Autodesk Inventor part; units mm, degrees
ref_plane "Work Plane8" through (0, 26.3, 0) normal (0, 1, 0) x (1, 0, 0)
ref_plane "Work Plane9" through (0, 30.1, 0) normal (0, 1, 0) x (1, 0, 0)
ref_plane "Work Plane15" through (-1.25, 15.4, 2.1651) normal (-0.5, 0, 0.866) x (0, -1, 0)
sketch "Sketch1" plane through (0, 0, 0) normal (1, 0, 0) x (0, 1, 0)
  line L0 (32, 0) -> (32, 2.45)
  line L1 (32, 2.45) -> (30.5, 2.45)
  line L2 (30.5, 2.45) -> (30.5, 2.125)
  line L3 (30.5, 2.125) -> (29.7, 2.125)
  line L4 (29.7, 2.125) -> (29.7, 2.45)
  line L5 (29.7, 2.45) -> (26.7, 2.45)
  line L6 (26.7, 2.45) -> (26.7, 2.125)
  line L7 (26.7, 2.125) -> (25.9, 2.125)
  line L8 (25.9, 2.125) -> (25.9, 2.45)
  line L9 (25.9, 2.45) -> (24.4, 2.45)
  line L10 (23.4, 2.5) -> (24.4, 2.5)
  line L11 (24.4, 2.5) -> (24.4, 2.45)
  line L12 (23.4, 2.5) -> (23.4, 7.5)
  line L13 (32, 2.45) -> (31, 2.45)
  line L14 (32, 2.45) -> (32, 1.45)
  line L15 (23.4, 7.5) -> (15.4, 7.5)
  line L16 (15.4, 7.5) -> (15.4, 0)
  line L17 (32, 0) -> (15.4, 0)
  point P0 (0, 0)
  dimension "d345" = 1.5
  dimension "d346" = 0.325
  dimension "d347" = 0.8
  dimension "d348" = 3
  dimension "d349" = 0.325
  dimension "d350" = 0.8
  dimension "d353" = 1
  dimension "d354" = 1
  dimension "d355" = 1
  dimension "d401" = 8
  dimension "d402" = 16.6
revolve "Revolution1" add sketch "Sketch1" angle 360 about axis through (0, 32, 0) along (0, -1, 0)
chamfer "Chamfer8" distance 1 angle 45 1 edges at (0, 32, -2.45)
sketch "Sketch13" plane through (0, 32, 0) normal (0, 1, 0) x (1, 0, 0)
  circle A0 centre (0, 0) radius 1
  point P0 (0, 0)
  dimension "d359" = 2
hole "Hole10" at (0, 32, 0) direction (0, -1, 0) diameter 2 end through all
ref_plane "Work Plane8" through (0, 26.3, 0) normal (0, 1, 0) x (1, 0, 0)
ref_plane "Work Plane9" through (0, 30.1, 0) normal (0, 1, 0) x (1, 0, 0)
sketch "Sketch16" plane through (0, 15.4, 0) normal (0, -1, 0) x (1, 0, 0)
  circle A0 centre (0, 0) radius 2.55
  dimension "d404" = 5.1
hole "Hole12" at (0, 15.4, 0) direction (0, 1, 0) diameter 5.1 depth 5
sketch "Sketch19" plane through (0, 15.4, 0) normal (0, -1, 0) x (1, 0, 0)
  circle A0 centre (0, 0) radius 7.5
  line L0 (0, 0) -> (7.5, 0)
  line L1 (0, 0) -> (-3.75, -6.4952)
  line L2 (0, 0) -> (7.5, 0) construction
  line L3 (0, 0) -> (-3.75, 6.4952)
  line L4 (0, 0) -> (7.5, 0) construction
  point P0 (0, 0)
  dimension "d423" = 7.5
  dimension "d424" = 120
  dimension "d425" = 7.5
  dimension "d426" = 120
ref_plane "Work Plane12" through (7.5, 15.4, 0) normal (1, 0, 0) x (0, 1, 0)
ref_plane "Work Plane13" through (-3.75, 15.4, 6.4952) normal (-0.5, 0, 0.866) x (0, -1, 0)
ref_plane "Work Plane14" through (-3.75, 15.4, -6.4952) normal (-0.5, 0, -0.866) x (0, -1, 0)
sketch "Sketch20" plane through (-3.75, 15.4, -6.4952) normal (-0.5, 0, -0.866) x (0, -1, 0)
  line L0 (0, -7.5) -> (0, 7.5)
  line L1 (0, 0) -> (-2.5, 0)
  point P0 (15.4, 0)
  dimension "d427" = 2.5
sketch "Sketch21" plane through (-3.75, 15.4, 6.4952) normal (-0.5, 0, 0.866) x (0, -1, 0)
  line L0 (0, -7.5) -> (0, 7.5)
  line L1 (0, 0) -> (-2.5, 0)
  point P0 (15.4, 0)
  dimension "d428" = 2.5
sketch "Sketch22" plane through (7.5, 15.4, 0) normal (1, 0, 0) x (0, 1, 0)
  line L0 (0, 0) -> (2.5, 0)
  point P0 (-15.4, 0)
  dimension "d429" = 2.5
hole "Hole14" at (-3.75, 17.9, 6.4952) direction (0.5, 0, -0.866) diameter 1.9 depth 6
hole "Hole15" at (-3.75, 17.9, -6.4952) direction (0.5, 0, 0.866) diameter 1.9 depth 6
hole "Hole16" at (7.5, 17.9, 0) direction (-1, 0, 0) diameter 1.9 depth 6
thread "Thread25"
thread "Thread26"
thread "Thread27"
chamfer "Chamfer9" distance 0.5 angle 45 2 edges at (0, 23.4, -7.5) (0, 15.4, -7.5)
chamfer "Chamfer10" distance 0.2 angle 45 1 edges at (0, 15.4, 2.55)
ref_plane "Work Plane15" through (-1.25, 15.4, 2.1651) normal (-0.5, 0, 0.866) x (0, -1, 0)
ref_plane "Work Plane16" through (2.5, 15.4, 0) normal (1, 0, 0) x (0, 1, 0)
ref_plane "Work Plane17" through (-1.25, 15.4, -2.1651) normal (-0.5, 0, -0.866) x (0, -1, 0)
properties part number "None_Magnet_Extender_Split_Top" material "Aluminum 6061"
Design review of the part built by this model. Coordinates are the model's own, in mm. A direction names the side the tool comes from. Give positions to 0.01 mm unless a question says otherwise; leave off trailing zeros. Write each loop counter-clockwise with the first axis right and the second up, starting at its lowest first coordinate (ties: lowest second). Pieces come first, ordered by that corner, then holes. Notation, with made-up numbers: M -1,65 L 5,65 A11 ccw 5,80 Z; hole C 65.25,77 d3. An arc over 180 degrees is marked long. Return JSON: item names as keys, results as strings. Group by question number.
Item 1: Take a section at D-D (y = 20). Give the boundary of the cut face in (x, z).
Item 2: Clearance check with flat-ended pins moving along their axes: pin 1 Ø1 at (x, y) = (-3, 23) entering from -Z; pin 2 Ø3 at (x, z) = (0, 6) entering from +Y; pin 3 Ø5.5 at (x, z) = (1.5, 0) entering from -Y; pin 4 Ø1.5 at (x, z) = (-1, 0) entering from -Y. State where each tip first meets the part, or that it passes through.
Item 3: The part is to be moulded in two halves that separate along X. For faces 4 (the flat face through (1, 20.4, -1)), 5 (the cylindrical face through (-1.792, 30.094, 1.142)), 6 (the cylindrical face through (4.897, 18.827, 0.206)), say which applies: pulls with the +X half, pulls with the -X half, needs draft (parallel to the pull), parting line crosses it, or undercut.
Item 4: Take a section at B-B (z = 0). Count the separate pieces of the cut face and the enclosed holes in it, plus the area to 3 significant figures.
Item 5: Wall thickness on line 1 along Z through (x, y) = (0, 24.75); line 2 along Z through (x, y) = (0, 17.45): over which ranges is each line inside the solid? List them lowest first.
Item 6: Take a section at C-C (y = 27.25). Give the boundary of the cut face in (x, z), plus the area to 3 significant figures.
Item 7: Tool access review of faces 1 (the cylindrical face through (-0.33, 19.351, -7.493)), 2 (the cylindrical face through (2.4, 25.1, -0.5)), 3 (the cylindrical face through (-1.792, 26.294, 1.142)): name each direction out of +Z, -Z, +X, -X, +Y, -Y from which nothing blocks a thin tool from reaching the whole face with its end or side.
Item 8: Take a section at A-A (y = 17.9). Give the boundary of the cut face in (x, z), plus the area to 3 significant figures.
Return value:
{
 "1": {"outline": "C 0,0 d15; hole C 0,0 d5.1"},
 "2": {"pin 1": "stops at z = -7.07", "pin 2": "stops at y = 23.4", "pin 3": "stops at y = 15.4", "pin 4": "stops at y = 20.4"},
 "3": {"face 4": "undercut", "face 5": "parting line crosses it", "face 6": "needs draft"},
 "4": {"separate pieces": "3", "enclosed holes": "0", "area": "102 mm2"},
 "5": {"line 1": "z = -2.45 to -1, 1 to 2.45", "line 2": "z = -7.5 to -2.55, 2.55 to 7.5"},
 "6": {"outline": "C 0,0 d4.9; hole C 0,0 d2", "area": "15.7 mm2"},
 "7": {"face 1": "+Y, -Y", "face 2": "+Y", "face 3": "none"},
 "8": {"outline": "M -4.54,-5.97 L -2.01,-1.57 A2.55 cw -2.01,1.57 L -4.54,5.97 A7.5 ccw Z; M -2.9,-6.92 A7.5 ccw 7.44,-0.95 L 2.37,-0.95 A2.55 cw -0.36,-2.52 Z; M -2.9,6.92 L -0.36,2.52 A2.55 cw 2.37,0.95 L 7.44,0.95 A7.5 ccw Z", "area": "128 mm2"}
}
